```python
from build123d import *

# Parameters (mm, degrees)
SKETCH1_W           = 69
SKETCH1_H           = 76.6
BOSS_EXTRUDE1_DEPTH = 1
SKETCH2_W           = 15
SKETCH2_H           = 15
BOSS_EXTRUDE2_DEPTH = 0.5
FILLET1_R           = 0.5


with BuildPart() as part:
    # Sketch1 → Boss-Extrude1 (new body)
    with BuildSketch(Plane(origin=(0, 0, 0), x_dir=(1, 0, 0), z_dir=(0, 1, 0))):
        Rectangle(SKETCH1_W, SKETCH1_H)
    extrude(amount=BOSS_EXTRUDE1_DEPTH)

    # Sketch2 → Boss-Extrude2 (add)
    with BuildSketch(Plane(origin=(0, 1, 0), x_dir=(1, 0, 0), z_dir=(0, 1, 0))):
        with Locations((-17, 8.8)):
            Rectangle(SKETCH2_W, SKETCH2_H)
        with Locations((-17, 25.8)):
            Rectangle(SKETCH2_W, SKETCH2_H)
        with Locations((0, 25.8)):
            Rectangle(SKETCH2_W, SKETCH2_H)
        with Locations((17, 25.8)):
            Rectangle(SKETCH2_W, SKETCH2_H)
        with Locations((0, 8.8)):
            Rectangle(SKETCH2_W, SKETCH2_H)
        with Locations((17, 8.8)):
            Rectangle(SKETCH2_W, SKETCH2_H)
        with Locations((-17, -8.2)):
            Rectangle(SKETCH2_W, SKETCH2_H)
        with Locations((0, -8.2)):
            Rectangle(SKETCH2_W, SKETCH2_H)
        with Locations((17, -8.2)):
            Rectangle(SKETCH2_W, SKETCH2_H)
        with Locations((-17, -25.2)):
            Rectangle(SKETCH2_W, SKETCH2_H)
        with Locations((0, -25.2)):
            Rectangle(SKETCH2_W, SKETCH2_H)
        with Locations((17, -25.2)):
            Rectangle(SKETCH2_W, SKETCH2_H)
    extrude(amount=BOSS_EXTRUDE2_DEPTH)

    # Fillet1
    fillet1_edges = [part.edges().sort_by_distance(p)[0] for p in [
        (17, 1, 32.7),
        (24.5, 1, 25.2),
        (17, 1, 17.7),
        (9.5, 1, 25.2),
        (-17, 1, 32.7),
        (-9.5, 1, 25.2),
        (-17, 1, 17.7),
        (-24.5, 1, 25.2),
        (0, 1, 15.7),
        (7.5, 1, 8.2),
        (0, 1, 0.7),
        (-7.5, 1, 8.2),
        (17, 1, -1.3),
        (24.5, 1, -8.8),
        (17, 1, -16.3),
        (9.5, 1, -8.8),
        (-17, 1, -1.3),
        (-9.5, 1, -8.8),
        (-17, 1, -16.3),
        (-24.5, 1, -8.8),
        (0, 1, -18.3),
        (7.5, 1, -25.8),
        (0, 1, -33.3),
        (-7.5, 1, -25.8),
        (34.5, 1, 0),
        (0, 1, 38.3),
        (-34.5, 1, 0),
        (0, 1, -38.3),
        (-17, 1, -18.3),
        (-9.5, 1, -25.8),
        (-17, 1, -33.3),
        (-24.5, 1, -25.8),
        (17, 1, -18.3),
        (24.5, 1, -25.8),
        (17, 1, -33.3),
        (9.5, 1, -25.8),
        (0, 1, -1.3),
        (7.5, 1, -8.8),
        (0, 1, -16.3),
        (-7.5, 1, -8.8),
        (-17, 1, 15.7),
        (-9.5, 1, 8.2),
        (-17, 1, 0.7),
        (-24.5, 1, 8.2),
        (17, 1, 15.7),
        (24.5, 1, 8.2),
        (17, 1, 0.7),
        (9.5, 1, 8.2),
        (0, 1, 32.7),
        (7.5, 1, 25.2),
        (0, 1, 17.7),
        (-7.5, 1, 25.2),
    ]]
    fillet(fillet1_edges, radius=FILLET1_R - 0.0001)  # a hair under: the kernel refuses the full size


solid = part.part
```
Design review of the part built by this model. Coordinates are the model's own, in mm. A direction names the side the tool comes from. Round coordinates to 2 decimals unless told otherwise and drop trailing zeros. Write each loop counter-clockwise with the first axis right and the second up, starting at its lowest first coordinate (ties: lowest second). Pieces come first, ordered by that corner, then holes. Notation, with made-up numbers: (31.25, 47.5) -> (41.25, 47.5) arc R28 cw to (41.25, 72.5) -> close; hole circle Ø3 at (55.5, 6.25). An arc over 180 degrees is marked (long way). Answer in a Markdown table with one row per item.
Q1. Take a section at B-B, the plane x = 29.5. State the section outline as (y, z) points.
The answers:
| item | result |
|---|---|
| outline | (0, -38.3) -> (0.5, -38.3) arc R0.5 ccw to (1, -37.8) -> (1, 37.8) arc R0.5 ccw to (0.5, 38.3) -> (0, 38.3) -> close |
Q2. Clearance check with flat-ended pins moving along their axes: pin 1 Ø4 at (x, z) = (26.5, 22) entering from -Y; pin 2 Ø1.5 at (x, z) = (26, 8.5) entering from +Y. State where each tip first meets the part, or that it passes through.
The answers:
| item | result |
|---|---|
| pin 1 | y = 0 |
| pin 2 | y = 1 |
Q3. To check wall thickness, follow L1, parallel to X at y = 1.4, z = -14; L2, parallel to Z at x = -11.5, y = 1.2; L3, parallel to Z at x = -17, y = 1.4. State the ranges of each line that lie inside material, in increasing order. Write a range as [from, to].
The answers:
| item | result |
|---|---|
| L1 | [-24.51, -9.49], [-7.51, 7.51], [9.49, 24.51] |
| L2 | [-33.4, -18.2], [-16.4, -1.2], [0.6, 15.8], [17.6, 32.8] |
| L3 | [-33.31, -18.29], [-16.31, -1.29], [0.69, 15.71], [17.69, 32.71] |
Q4. For faces 1 (the face through (17, 1.5, 8)), 2 (the face through (-0.5, 1, -0.5)), list the 3-axis set-ups (+Z, -Z, +X, -X, +Y, -Y) from which the entire face can be reached by the end or side of a thin tool; tool diameter is ignored.
The answers:
| item | result |
|---|---|
| face 1 | +Z, -Z, +X, -X, +Y |
| face 2 | +Y |
